For this review, take the finished solid that the model builds, in its own axes (mm). Round coordinates to 2 decimals unless told otherwise and drop trailing zeros. Write each loop counter-clockwise with the first axis right and the second up, starting at its lowest first coordinate (ties: lowest second). Pieces come first, ordered by that corner, then holes. Notation, with made-up numbers: (-4, 33.25) - (39, 33.25) arc R28 ccw to (39, 70.25) - close; hole circle Ø9 at (35.5, 11). An arc over 180 degrees is marked (long way). One line per item, written item: value. Start each with the question number.
Q1. Add section C-C on x = 0.75. Write out the cut boundary in (y, z).
Q2. Clearance check with flat-ended pins moving along their axes: pin 1 Ø5 at (y, z) = (0, 0) entering from -X; pin 2 Ø1.5 at (x, y) = (-1.5, -3.5) entering from +Z. State where each tip first meets the part, or that it passes through.
Q3. Mouldability with a two-part tool opening along X and no side actions: class faces 1 (the face through (-0.01, 7.81, -1.73)), 2 (the face through (-2.3, 2, 0)), 3 (the face through (0.03, -0.45, 1.43)), 4 (the face through (2.3, 2, 0)) as +X half, -X half, draft (parallel to the pull), parting line (faces both ways), or undercut.
Q4. For probe 1 along Y at (x, z) = (-0.9, 0); probe 2 along X at (y, z) = (3, -8); probe 3 along Y at (x, z) = (1.8, 4.25), list the stretches that pass through material, from the lowest coordinate up.
```python
from build123d import *

# Parameters (mm, degrees)
FILLET1_R = 0.5


with BuildPart() as part:
    # Sketch1 → Revolve1 (revolve)
    with BuildSketch(Plane.XY, mode=Mode.PRIVATE) as revolve1_sk:
        with BuildLine():
            Line((-2.3, 1.5), (2.3, 1.5))
            Line((2.3, 1.5), (2.3, 9))
            Line((2.3, 9), (1.55, 9))
            Line((1.55, 9), (1.55, 8.5))
            ThreePointArc((1.55, 8.5), (1.403553391, 8.146446609), (1.05, 8))
            Line((1.05, 8), (-1.05, 8))
            ThreePointArc((-1.05, 8), (-1.403553391, 8.146446609), (-1.55, 8.5))
            Line((-1.55, 8.5), (-1.55, 9))
            Line((-1.55, 9), (-2.3, 9))
            Line((-2.3, 9), (-2.3, 1.5))
        make_face()
    revolve(revolve1_sk.sketch.rotate(Axis((0, 0, 0), (1, 0, 0)), 90), axis=Axis((0, 0, 0), (1, 0, 0)))

    # Fillet1
    fillet1_edges = [part.edges().sort_by_distance(p)[0] for p in [
        (1.55, 0, -9),
        (-1.55, 0, -9),
    ]]
    fillet(fillet1_edges, radius=FILLET1_R - 0.0001)  # a hair under: the kernel refuses the full size


solid = part.part
```
Result set:
1. outline: circle Ø16 at (0, 0); hole circle Ø3 at (0, 0)
2. pin 1: stops at x = -2.3
2. pin 2: stops at z = 8.51
3. face 1: undercut
3. face 2: -X half
3. face 3: draft
3. face 4: +X half
4. probe 1: y = -8 to -1.5, 1.5 to 8
4. probe 2: x = -2.3 to -1.55, 1.55 to 2.3
4. probe 3: y = -7.86 to 7.86
